from build123d import *

# Parameters (mm, degrees)
BOSS_EXTRUDE1_DEPTH      = 22
CUT_EXTRUDE1_DEPTH       = 40.705228033
CUT_EXTRUDE1_DEPTH_BACK  = 40.705228033
BOSS_EXTRUDE2_DEPTH      = 8
BOSS_EXTRUDE2_DEPTH_BACK = 8


with BuildPart() as part:
    # Sketch1 → Boss-Extrude1 (new body)
    with BuildSketch(Plane(origin=(0, 0, 0), x_dir=(1, 0, 0), z_dir=(0, 1, 0))):
        Polygon((-27.721925134, 18), (-27.721925134, -18), (7.278074866, -8), (7.278074866, 8), align=None)
    extrude(amount=BOSS_EXTRUDE1_DEPTH)

    # Sketch2 → Cut-Extrude1 (cut, two sides: drawn at the far end of the back side and taken through both)
    with BuildSketch(Plane.XY.offset(-CUT_EXTRUDE1_DEPTH_BACK)):
        Polygon((-9.721925134, 14), (-9.721925134, 8), (7.278074866, 5), (7.278074866, 17), align=None)
    extrude(amount=CUT_EXTRUDE1_DEPTH + CUT_EXTRUDE1_DEPTH_BACK, mode=Mode.SUBTRACT)

    # Sketch3 → Boss-Extrude2 (add, two sides: drawn at the far end of the back side and taken through both)
    with BuildSketch(Plane.XY.offset(-BOSS_EXTRUDE2_DEPTH_BACK)):
        Polygon((-39.721925134, 30), (-39.721925134, -8), (-17.721925134, -8), (-17.721925134, 0), (-27.721925134, 0), (-27.721925134, 22), (-17.721925134, 22), (-17.721925134, 30), align=None)
    extrude(amount=BOSS_EXTRUDE2_DEPTH + BOSS_EXTRUDE2_DEPTH_BACK)


solid = part.part
Design review of the part built by this model. Coordinates are the model's own, in mm. A direction names the side the tool comes from. Give positions to 0.01 mm unless a question says otherwise; leave off trailing zeros. Order: outer loops, then holes, each group sorted by start corner. A loop starts at its lowest first (then second) coordinate and runs counter-clockwise, first axis right, second up.
1. Add section B-B, the plane x = -1.5. State the section outline as (y, z) points, then the cut area to 3 significant figures.
Solution:
outline: (0, -10.51) - (6.55, -10.51) - (6.55, 10.51) - (0, 10.51) - close; (15.45, -10.51) - (22, -10.51) - (22, 10.51) - (15.45, 10.51) - close
area: 275 mm2
2. Add section C-C, the plane z = 3.5. State the section outline as (x, y) points, then the cut area to 3 significant figures.
Solution:
outline: (-39.72, -8) - (-17.72, -8) - (-17.72, 0) - (7.28, 0) - (7.28, 5) - (-9.72, 8) - (-9.72, 14) - (7.28, 17) - (7.28, 22) - (-17.72, 22) - (-17.72, 30) - (-39.72, 30) - close
area: 1,230 mm2
3. Mouldability with a two-part tool opening along Y and no side actions: class faces 6 (the flat face through (-1.1, 15.52, -0.18)), 7 (the flat face through (7.278, 19, 0)), 8 (the flat face through (-29, -8, 0)) as +Y half, -Y half, draft (parallel to the pull), parting line (faces both ways), or undercut.
Solution:
face 6: undercut
face 7: draft
face 8: -Y half
4. Add section A-A, the plane y = 1. State the section outline as (x, z) points.
Solution:
outline: (-39.72, -8) - (-27.72, -8) - (-27.72, -18) - (7.28, -8) - (7.28, 8) - (-27.72, 18) - (-27.72, 8) - (-39.72, 8) - close
5. For pin 1 Ø12 at (x, y) = (-16, 2.5) entering from +Z; pin 2 Ø1.5 at (x, z) = (-18, 9.5) entering from -Y; pin 3 Ø5 at (y, z) = (7, -15) entering from -X, all flat-tipped, find the tip position at first contact; note any pin that passes through.
Solution:
pin 1: stops at z = 16.37
pin 2: stops at y = 0
pin 3: stops at x = -27.72
6. Add section D-D, the plane x = -26. State the section outline as (y, z) points, then the cut area to 3 significant figures.
Solution:
outline: (-8, -8) - (0, -8) - (0, -17.51) - (22, -17.51) - (22, -8) - (30, -8) - (30, 8) - (22, 8) - (22, 17.51) - (0, 17.51) - (0, 8) - (-8, 8) - close
area: 1,030 mm2
7. Tool access review of faces 1 (the flat face through (-9.722, 11, 0)), 2 (the flat face through (-17.722, -4, 0)), 3 (the flat face through (-17.722, 26, 0)), 4 (the flat face through (-27.722, 11, 13)), 5 (the flat face through (-27.722, 11, -13)): name each direction out of +Z, -Z, +X, -X, +Y, -Y from which nothing blocks a thin tool from reaching the whole face with its end or side.
Solution:
face 1: +Z, -Z, +X
face 2: +Z, -Z, +X, -Y
face 3: +Z, -Z, +X, +Y
face 4: +Z, -X, +Y, -Y
face 5: -Z, -X, +Y, -Y
8. To check wall thickness, follow L1, parallel to Z at x = -37.5, y = 13.5; L2, parallel to Y at x = -23.5, z = -14.5; L3, parallel to X at y = 13.5, z = 4.5. State the ranges of each line that lie inside material, in increasing order.
Solution:
L1: z = -8 to 8
L2: y = 0 to 22
L3: x = -39.72 to -9.72
